Could you check a few things on this model? Use its own coordinates, in mm. Face numbers are marked on the shaded views. A direction names the side the tool comes from. Give positions to 0.01 mm unless a question says otherwise; leave off trailing zeros. Write each loop counter-clockwise with the first axis right and the second up, starting at its lowest first coordinate (ties: lowest second). Pieces come first, ordered by that corner, then holes. Notation, with made-up numbers: (-22, -3) - (18, -3) arc R27 ccw to (18, 17) - close; hole circle Ø5 at (-1.75, 22.25). An arc over 180 degrees is marked (long way). Answer in a Markdown table with one row per item.
from build123d import *

# Parameters (mm, degrees)
F0_W      = 30
F0_H      = 30
F1_DEPTH  = 25
F6_W      = 15
F6_H      = 20
F10_DEPTH = 5
F11_DEPTH = 30.0010001
F12_DEPTH = 15


with BuildPart() as f1:
    # F0 (on Top) → F1 (new body)
    with BuildSketch(Plane.XY):
        with Locations((15, 15)):
            Rectangle(F0_W, F0_H)
    extrude(amount=F1_DEPTH)

    # F2 (on face) → F7 section 0
    with BuildSketch(Plane.XY.offset(25), mode=Mode.PRIVATE) as f7_s0:
        Polygon((0, 10), (20, 30), (0, 30), align=None)
    loft([f7_s0.sketch, Vertex(0, 10, 5)], mode=Mode.SUBTRACT)

    # F2 (on face) → F8 section 0
    with BuildSketch(Plane.XY.offset(25), mode=Mode.PRIVATE) as f8_s0:
        Polygon((30, 0), (30, 30), (20, 20), align=None)
    loft([f8_s0.sketch, Vertex(30, 0, 5)], mode=Mode.SUBTRACT)

    # F3 (on face) → F9 section 0
    with BuildSketch(Plane.XZ, mode=Mode.PRIVATE) as f9_s0:
        Polygon((30, 25), (20, 25), (30, 5), align=None)
    loft([f9_s0.sketch, Vertex(20, 20, 25)], mode=Mode.SUBTRACT)

    # F6 (on face) → F10 (cut)
    with BuildSketch(Plane(origin=(0, 0, 0), x_dir=(1, 0, 0), z_dir=(0, 0, -1))):
        with Locations((17.5, -10)):
            Rectangle(F6_W, F6_H)
    extrude(amount=-F10_DEPTH, mode=Mode.SUBTRACT)

    # F4 (on face) → F11 (cut, through all)
    with BuildSketch(Plane.YZ.offset(30)):
        Polygon((0, 25), (0, 5), (20, 25), align=None)
    extrude(amount=-F11_DEPTH, mode=Mode.SUBTRACT)

    # F2 (on face) → F12 (cut)
    with BuildSketch(Plane.XY.offset(25)):
        Polygon((30, 30), (20, 30), (0, 10), (0, 0), (20, 20), align=None)
    extrude(amount=-F12_DEPTH, mode=Mode.SUBTRACT)

    # F13 (on face) → F14 (join, up to the next surface of F1)
    with BuildSketch(Plane.XZ):
        Polygon((0, 5), (5, 10), (0, 10), align=None)
    extrude(until=Until.NEXT, dir=(0, 1, 0))


solid = f1.part
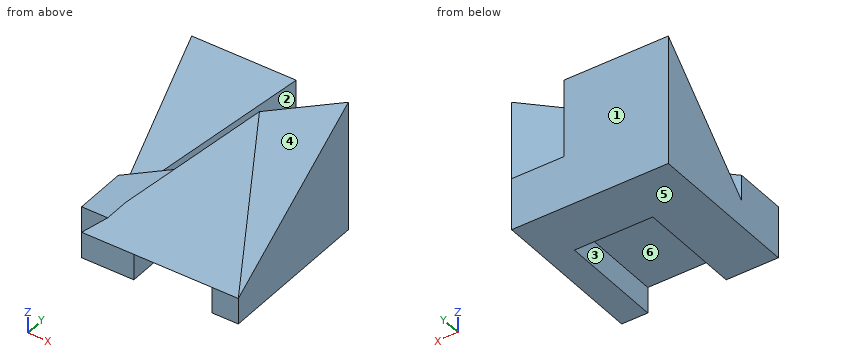
1) Imagine slicing it at D-D (z = 8.5). List the corners of the cut face in (x, y) for me.
Check values:
| item | result |
|---|---|
| outline | (0, 0) - (3.5, 0) - (3.5, 3.5) - (28.25, 3.5) - (30, 5.25) - (30, 30) - (0, 30) - (0, 13.5) - (3.5, 13.5) - (0, 10) - close |
2) We'd pull the mould along X, two halves only. Please class the marked faces 4, 5 and 6: +X half, -X half, draft (parallel to the pull), parting line (faces both ways), or undercut.
Check values:
| item | result |
|---|---|
| face 4 | +X half |
| face 5 | draft |
| face 6 | undercut |
3) Imagine slicing it at A-A (z = 21.5). List the corners of the cut face in (x, y) for me.
Check values:
| item | result |
|---|---|
| outline | (0, 26.5) - (16.5, 26.5) - (20, 30) - (0, 30) - close; (16.5, 16.5) - (21.75, 16.5) - (30, 24.75) - (30, 30) - close |
4) If I drill on line 1 (X direction, y = 10, z = 3.5); line 2 (Z direction, x = 6, y = 14.5); line 3 (Y direction, x = 23, z = 2.25), over which ranges is the centre line in solid material (lowest first)?
Check values:
| item | result |
|---|---|
| line 1 | x = 0 to 10, 25 to 30 |
| line 2 | z = 0 to 10 |
| line 3 | y = 20 to 30 |
5) On a 3-axis mill with a long thin cutter (end or side, diameter ignored), from which of +Z, -Z, +X, -X, +Y, -Y can I reach the whole of each face in a straight line? I mean the marked faces 1, 2 and 3. Say none if no direction works.
Check values:
| item | result |
|---|---|
| face 1 | +Z, -Z, +X, -X, +Y |
| face 2 | +Z |
| face 3 | -Z, -Y |
6) Imagine slicing it at B-B (x = 26.5). List the corners of the cut face in (y, z) for me.
Check values:
| item | result |
|---|---|
| outline | (0, 0) - (30, 0) - (30, 10) - (26.5, 10) - (26.5, 25) - (7, 12) - (0, 5) - close |
7) Imagine slicing it at C-C (y = 25.5). List the corners of the cut face in (x, z) for me.
Check values:
| item | result |
|---|---|
| outline | (0, 0) - (30, 0) - (30, 22) - (25.5, 25) - (25.5, 10) - (15.5, 10) - (15.5, 20.5) - (0, 20.5) - close |
8) Will these pins go through, and if not, where does the flat tip stop? P1, Ø4, axis at x = 17, y = 6, coming from the -Z side; P2, Ø8, axis at x = 18.5, z = 19.5, coming from the -Y side; P3, Ø2.5, axis at x = 20.5, z = 2.5, coming from the -Y side.
Check values:
| item | result |
|---|---|
| P1 | stops at z = 5 |
| P2 | stops at y = 10.5 |
| P3 | stops at y = 20 |
